Input: part model. Units: mm. Frame: model coordinates. A direction names the side the tool comes from. Round coordinates to 2 decimals unless told otherwise and drop trailing zeros. Loops run counter-clockwise (first coordinate to the right, second up) from the corner with the lowest first, then second, coordinate; pieces in that order, holes last. Notation, with made-up numbers: (-33.75, 55) -> (6.25, 55) arc R19 cw to (6.25, 66) -> close; hole circle Ø1 at (54.5, 35.5). An arc over 180 degrees is marked (long way). Answer as a JSON object with one key per item and string values.
Autodesk Inventor part; units mm, degrees
ref_plane "YZ Plane" through (0, 0, 0) normal (1, 0, 0) x (0, 1, 0)
ref_plane "XZ Plane" through (0, 0, 0) normal (0, 1, 0) x (-1, 0, 0)
ref_plane "XY Plane" through (0, 0, 0) normal (0, 0, 1) x (1, 0, 0)
sketch "Sketch1" plane through (0, 0, 0) normal (0, 0, 1) x (1, 0, 0)
  line L0 (-1.75, -53.75) -> (-1.75, 11.25)
  line L1 (35.25, -53.75) -> (-1.75, -53.75)
  line L2 (35.25, 11.25) -> (35.25, -53.75)
  line L3 (-1.75, 11.25) -> (35.25, 11.25)
  circle A0 centre (30, 8) radius 3
  circle A1 centre (3.5, -50.5) radius 3
  circle A2 centre (30, -50.5) radius 3
  circle A3 centre (3.5, 8) radius 3
  circle A4 centre (3.5, -50.5) radius 1.45
  circle A5 centre (30, -50.5) radius 1.45
  circle A6 centre (30, 8) radius 1.45
  circle A7 centre (3.5, 8) radius 1.45
  point P0 (0, 0)
  dimension "d0" = 2.9
  dimension "d1" = 2.9
  dimension "d2" = 2.9
  dimension "d3" = 2.9
extrude "Extrusion1" add sketch "Sketch1" along normal blind 3 contours L0 L3 L2 L1 | A0 | A1 | A2 | A3
sketch "Sketch2" plane through (0, 0, 0) normal (0, 0, -1) x (-1, 0, 0)
  line L0 (-35.25, -53.75) -> (-35.25, 11.25)
  line L1 (-35.25, 11.25) -> (-35.75, 11.25)
  line L2 (-35.75, 11.25) -> (-37.75, 11.25)
  line L3 (-37.75, 11.25) -> (-37.75, 11.75)
  line L4 (-37.75, 11.75) -> (-37.75, 13.75)
  line L5 (-37.75, 13.75) -> (1.75, 13.75)
  line L6 (1.75, 13.75) -> (2.25, 13.75)
  line L7 (2.25, 13.75) -> (4.25, 13.75)
  line L8 (4.25, 13.75) -> (4.25, -53.75)
  line L9 (4.25, -53.75) -> (4.25, -54.25)
  line L10 (4.25, -54.25) -> (4.25, -56.25)
  line L11 (4.25, -56.25) -> (-35.25, -56.25)
  line L12 (-35.25, -56.25) -> (-37.75, -56.25)
  line L13 (-37.75, -56.25) -> (-37.75, 11.25)
  line L14 (-37.75, 11.75) -> (4.25, 11.75)
  line L15 (1.75, 11.25) -> (1.75, -53.75)
  line L16 (1.75, 11.25) -> (1.75, 11.75)
  line L17 (2.25, 13.75) -> (2.25, -56.25)
  line L18 (1.75, -53.75) -> (4.25, -53.75)
  line L19 (4.25, -54.25) -> (-35.25, -54.25)
  line L20 (1.75, -53.75) -> (-35.25, -53.75)
  line L21 (-35.25, -54.25) -> (-37.75, -54.25)
  line L22 (-35.25, -53.75) -> (-35.25, -54.25)
  line L23 (-35.75, 11.25) -> (-35.75, -56.25)
  line L24 (-35.25, 11.25) -> (1.75, 11.25)
  line L25 (-35.75, 11.25) -> (-35.75, 13.75)
  point P0 (0, 0)
  point P1 (-35.75, -54.25)
  point P2 (-35.75, 11.75)
  point P3 (2.25, 11.75)
  point P4 (2.25, -54.25)
  dimension "d6" = 0.5
  dimension "d7" = 2
  dimension "d8" = 0.5
  dimension "d9" = 2
  dimension "d10" = 0.5
  dimension "d11" = 2
  dimension "d12" = 0.5
  dimension "d13" = 2
extrude "Extrusion2" add sketch "Sketch2" against normal up to surface (3 mm away) contours L22 L21 L23 L1 L0 | L20 L18 L17 L19 L22 | L1 L25 L14 L16 L24 | L15 L16 L14 L17 L18 | L19 L17 L11 L12 L23 L21 | L23 L21 L13 L2 | L2 L3 L14 L25 | L18 L9 L19 L17 | L17 L14 L8 L18 | L19 L10 L11 L17 | L23 L12 L13 L21 | L25 L5 L6 L17 L14 | L14 L4 L5 L25 | L17 L7 L8 L14
extrude "Extrusion3" add sketch "Sketch1" against normal blind 3 contours A0 | A1 | A2 | A3
extrude "Extrusion4" add sketch "Sketch2" along normal blind 4.5 contours L19 L17 L11 L12 L23 L21 | L23 L21 L13 L2 | L2 L3 L14 L25 | L18 L9 L19 L17 | L17 L14 L8 L18 | L19 L10 L11 L17 | L23 L12 L13 L21 | L25 L5 L6 L17 L14 | L14 L4 L5 L25 | L17 L7 L8 L14
sketch "Sketch3" plane through (0, 0, 0) normal (0, 0, -1) x (-1, 0, 0)
  line L0 (-35.75, 11.75) -> (2.25, 11.75)
  line L1 (-16.75, 11.75) -> (-16.75, -54.25)
  line L2 (2.25, -54.25) -> (-35.75, -54.25)
  circle A0 centre (-16.75, -6.3689) radius 1.45
  circle A1 centre (-16.75, -6.3689) radius 3
  line L3 (-16.75, -6.3689) -> (-16.75, -36.3689)
  circle A2 centre (-16.75, -36.3689) radius 1.45
  circle A3 centre (-16.75, -36.3689) radius 3
  point P0 (0, 0)
  dimension "d20" = 2.9
  dimension "d21" = 6
  dimension "d22" = 30
  dimension "d23" = 2.9
  dimension "d24" = 6
extrude "Extrusion5" cut sketch "Sketch3" against normal up to surface (3 mm away) contours A0 L1 | L1 A0 | A2 L1 | L1 A2
extrude "Extrusion6" cut sketch "Sketch3" against normal blind 1 contours A1 L1 A0 | L1 A0 A1 | A3 L1 A2 | L1 A2 A3
sketch "Sketch4" plane through (0, 0, 0) normal (0, 0, -1) x (-1, 0, 0)
  circle A0 centre (-16.75, -16.3009) radius 4.767
  point P0 (0, 0)
  point P1 (-16.75, -6.3689)
  dimension "d30" = 9.534
extrude "Extrusion7" cut sketch "Sketch4" against normal up to surface (3 mm away)
equation "\"d14\" = d7"
properties part number "converter_case"
1) Draft query along Y for faces 3 (the face through (17, 13.75, -1)), 4 (the face through (27, 8, -1)), 5 (the face through (37.75, -22, -1)), 6 (the face through (31.38, -50.94, -0.04)). Return one class per face: +Y half, -Y half, draft (parallel to the pull), parting line (faces both ways), or undercut.
Output:
{"face 3": "+Y half", "face 4": "undercut", "face 5": "draft", "face 6": "undercut"}
2) Section B-B, the plane x = 30. Output: boundary loops of the cut face in (y, z), plus the area to 3 significant figures.
Output:
{"outline": "(-56.25, -4.5) -> (-54.25, -4.5) -> (-54.25, 0) -> (-53.5, 0) -> (-53.5, -3) -> (-51.95, -3) -> (-51.95, 3) -> (-56.25, 3) -> close; (-49.05, -3) -> (-47.5, -3) -> (-47.5, 0) -> (5, 0) -> (5, -3) -> (6.55, -3) -> (6.55, 3) -> (-49.05, 3) -> close; (9.45, -3) -> (11, -3) -> (11, 0) -> (11.75, 0) -> (11.75, -4.5) -> (13.75, -4.5) -> (13.75, 3) -> (9.45, 3) -> close", "area": "229 mm^2"}
3) Ray query, probe 1 along Y at (x, z) = (30, 1.4); probe 2 along Y at (x, z) = (16.75, 2.2); probe 3 along Y at (x, z) = (3.5, -0.9). Return the intervals inside material, ascending.
Output:
{"probe 1": "y = -56.25 to -51.95, -49.05 to 6.55, 9.45 to 13.75", "probe 2": "y = -56.25 to -37.82, -34.92 to -21.07, -11.53 to -7.82, -4.92 to 13.75", "probe 3": "y = -56.25 to -54.25, -53.5 to -51.95, -49.05 to -47.5, 5 to 6.55, 9.45 to 11, 11.75 to 13.75"}
4) Section A-A, the plane z = -2.25. Count the separate pieces of the cut face and the enclosed holes in it, plus the area to 3 significant figures.
Output:
{"separate pieces": "5", "enclosed holes": "5", "area": "519 mm^2"}
5) Contact query for flat-ended pins moving along their axis: P1, Ø3, axis at x = 6, y = -17, coming from the -Z side; P2, Ø5, axis at x = 3.5, y = -51.5, coming from the -Z side. Output: stop coordinate, or through.
Output:
{"P1": "stops at z = 0", "P2": "stops at z = -3"}
6) Section C-C, the plane y = -50.5. Output: boundary loops of the cut face in (x, z), plus the area to 3 significant figures.
Output:
{"outline": "(-4.25, -4.5) -> (-2.25, -4.5) -> (-2.25, 0) -> (0.5, 0) -> (0.5, -3) -> (2.05, -3) -> (2.05, 3) -> (-4.25, 3) -> close; (4.95, -3) -> (6.5, -3) -> (6.5, 0) -> (27, 0) -> (27, -3) -> (28.55, -3) -> (28.55, 3) -> (4.95, 3) -> close; (31.45, -3) -> (33, -3) -> (33, 0) -> (35.75, 0) -> (35.75, -4.5) -> (37.75, -4.5) -> (37.75, 3) -> (31.45, 3) -> close", "area": "145 mm^2"}
7) Reachability of faces 1 (the face through (12, -21, 3)), 2 (the face through (29, -52, -3)) from +Z, -Z, +X, -X, +Y, -Y: full face, straight path, thin tool, end or side. Return the list, or none.
Output:
{"face 1": "+Z, +X, -X, +Y, -Y", "face 2": "-Z"}
8) Section D-D, the plane x = 16.75. Output: boundary loops of the cut face in (y, z).
Output:
{"outline": "(-56.25, -4.5) -> (-54.25, -4.5) -> (-54.25, 0) -> (-39.37, 0) -> (-39.37, 1) -> (-37.82, 1) -> (-37.82, 3) -> (-56.25, 3) -> close; (-34.92, 1) -> (-33.37, 1) -> (-33.37, 0) -> (-21.07, 0) -> (-21.07, 3) -> (-34.92, 3) -> close; (-11.53, 0) -> (-9.37, 0) -> (-9.37, 1) -> (-7.82, 1) -> (-7.82, 3) -> (-11.53, 3) -> close; (-4.92, 1) -> (-3.37, 1) -> (-3.37, 0) -> (11.75, 0) -> (11.75, -4.5) -> (13.75, -4.5) -> (13.75, 3) -> (-4.92, 3) -> close"}
